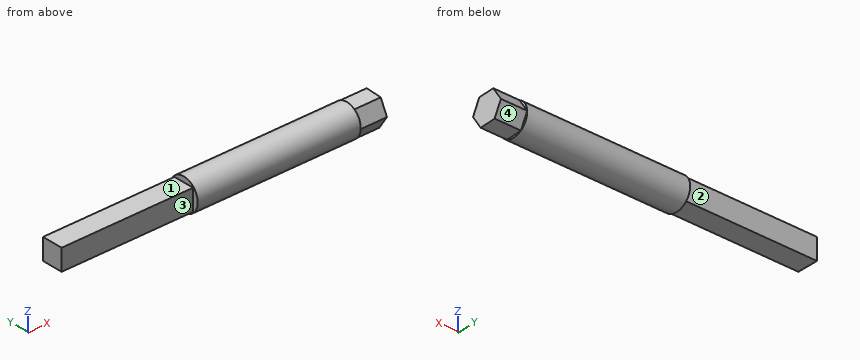
from build123d import *

# Parameters (mm, degrees)
SKETCH3_R           = 3
BOSS_EXTRUDE1_DEPTH = 31
BOSS_EXTRUDE4_DEPTH = 5
SKETCH18_W          = 4
SKETCH18_H          = 4
BOSS_EXTRUDE5_DEPTH = 30
SKETCH21_W          = 4
SKETCH21_H          = 4
CUT_EXTRUDE1_DEPTH  = 5


with BuildPart() as part:
    # Sketch1 → Loft1 section 0
    with BuildSketch(Plane(origin=(0, 0, 0), x_dir=(0, 0, -1), z_dir=(1, 0, 0))):
        with BuildLine():
            Line((-1, -1), (1, -1))
            Line((1, -1), (1, 1))
            Line((1, 1), (-1, 1))
            Line((-1, 1), (-1, -1))
        make_face()
    # Sketch2 → Loft1 section 1
    with BuildSketch(Plane(origin=(30, 0, 0), x_dir=(0, 0, -1), z_dir=(1, 0, 0))):
        with BuildLine():
            Line((-1, -1), (1, -1))
            Line((1, -1), (1, 1))
            Line((1, 1), (-1, 1))
            Line((-1, 1), (-1, -1))
        make_face()
    loft()

    # Sketch3 → Boss-Extrude1 (add)
    with BuildSketch(Plane(origin=(30, 0, 0), x_dir=(0, 0, -1), z_dir=(1, 0, 0))):
        Circle(SKETCH3_R)
    extrude(amount=BOSS_EXTRUDE1_DEPTH)

    # Sketch17 → Boss-Extrude4 (add)
    with BuildSketch(Plane(origin=(61, 0, 0), x_dir=(0, 0, -1), z_dir=(1, 0, 0))):
        Polygon((2.507905391, 1.646332454), (-0.171813033, 2.995076006), (-2.679718424, 1.348743552), (-2.507905391, -1.646332454), (0.171813033, -2.995076006), (2.679718424, -1.348743552), align=None)
    extrude(amount=BOSS_EXTRUDE4_DEPTH)

    # Sketch18 → Boss-Extrude5 (add)
    with BuildSketch(Plane.ZY):
        Rectangle(SKETCH18_W, SKETCH18_H)
    extrude(amount=-BOSS_EXTRUDE5_DEPTH)

    # Sketch21 → Cut-Extrude1 (cut)
    with BuildSketch(Plane.ZY):
        Rectangle(SKETCH21_W, SKETCH21_H)
    extrude(amount=-CUT_EXTRUDE1_DEPTH, mode=Mode.SUBTRACT)


solid = part.part
Part model, mm, in its own coordinate system. Face numbers are marked on the shaded views. A direction names the side the tool comes from. Give positions to 0.01 mm unless a question says otherwise; leave off trailing zeros. Loops run counter-clockwise (first coordinate to the right, second up) from the corner with the lowest first, then second, coordinate; pieces in that order, holes last.
(1) Band-saw the part on B-B (z = 0.75). Write the cut outline in (x, y), and give its area (3 significant figures).
Return value:
outline: (5, -2) - (30, -2) - (30, -2.9) - (61, -2.9) - (61, -2.53) - (66, -2.53) - (66, 2.62) - (61, 2.62) - (61, 2.9) - (30, 2.9) - (30, 2) - (5, 2) - close
area: 306 mm2
(2) Band-saw the part on C-C (x = 13.5). Write the cut outline in (y, z).
Return value:
outline: (-2, -2) - (2, -2) - (2, 2) - (-2, 2) - close
(3) Drill centre lines: line 1 along X through (y, z) = (-2.05, -0.6); line 2 along Z through (x, y) = (16, -0.15). Where is each one in solid material? Low to high.
Return value:
line 1: x = 30 to 66
line 2: z = -2 to 2
(4) 3-axis set-ups, long thin cutter, end or side, ignore diameter. For the marked faces 1, 2, 3 and 4: which of +Z, -Z, +X, -X, +Y, -Y reach the whole face in a straight line?
Return value:
face 1: +Z, -X, +Y, -Y
face 2: +Z, -Z, -X, +Y
face 3: +Z, -Z, -X, -Y
face 4: -Z, +X, +Y
(5) Band-saw the part on A-A (y = 0). Write the cut outline in (x, z).
Return value:
outline: (5, -2) - (30, -2) - (30, -3) - (61, -3) - (61, -2.6) - (66, -2.6) - (66, 2.6) - (61, 2.6) - (61, 3) - (30, 3) - (30, 2) - (5, 2) - close
(6) Band-saw the part on D-D (x = 52). Write the cut outline in (y, z).
Return value:
outline: circle Ø6 at (0, 0)
(7) Pin check, flat tips, straight feed: pin 1 (0.8 mm diameter, centred on y = 2.5, z = 2, fed in from +X); pin 2 (2 mm diameter, centred on x = 21, y = 0, fed in from +Z); pin 3 (1.5 mm diameter, centred on x = 26, z = 0, fed in from -Y). Stop position of each tip, or through.
Return value:
pin 1: stops at x = 61
pin 2: stops at z = 2
pin 3: stops at y = -2
